Input: dimensioned drawing with shaded views. Units: mm. Origin: part minimum x, y, z. Round coordinates to 2 decimals unless told otherwise and drop trailing zeros. Order: outer loops, then holes, each group sorted by start corner. A loop starts at its lowest first (then second) coordinate and runs counter-clockwise, first axis right, second up. Notation, with made-up numbers: M 31.5,65.25 L 54.5,65.25 A9 ccw 54.5,79.25 Z; hole C 43,63 d9. An arc over 180 degrees is marked long. Answer as CSV lines item,"result". Start each with the question number.
Item 1: Line query: line 1 (Z direction, x = 5, y = 2.3); line 2 (X direction, y = 2.95, z = 3); line 3 (X direction, y = 6.5, z = 2.25). Output: solid intervals per line, ascending. Write a range as [from, to].
Item 2: First-contact query: P1, Ø1, axis at y = 5, z = 2.5, coming from the +X side. Flat tip, straight axial feed; report the tip coordinate or a pass-through.
Item 3: Section query B-B on y = 5. Return the cut outline in (x, z), plus the area to 3 significant figures.
Item 4: Section query D-D on z = 0.45. Return the cut outline in (x, y).
Item 5: Pull-direction query (Z, two-part tool) for the marked faces 1, 2 and 3; classes: +Z half, -Z half, draft (parallel to the pull), parting line (faces both ways), or undercut.
Item 6: Section query A-A on z = 3. Return the cut outline in (x, y).
Item 7: Section query C-C on x = 7. Return the cut outline in (y, z), plus the area to 3 significant figures.
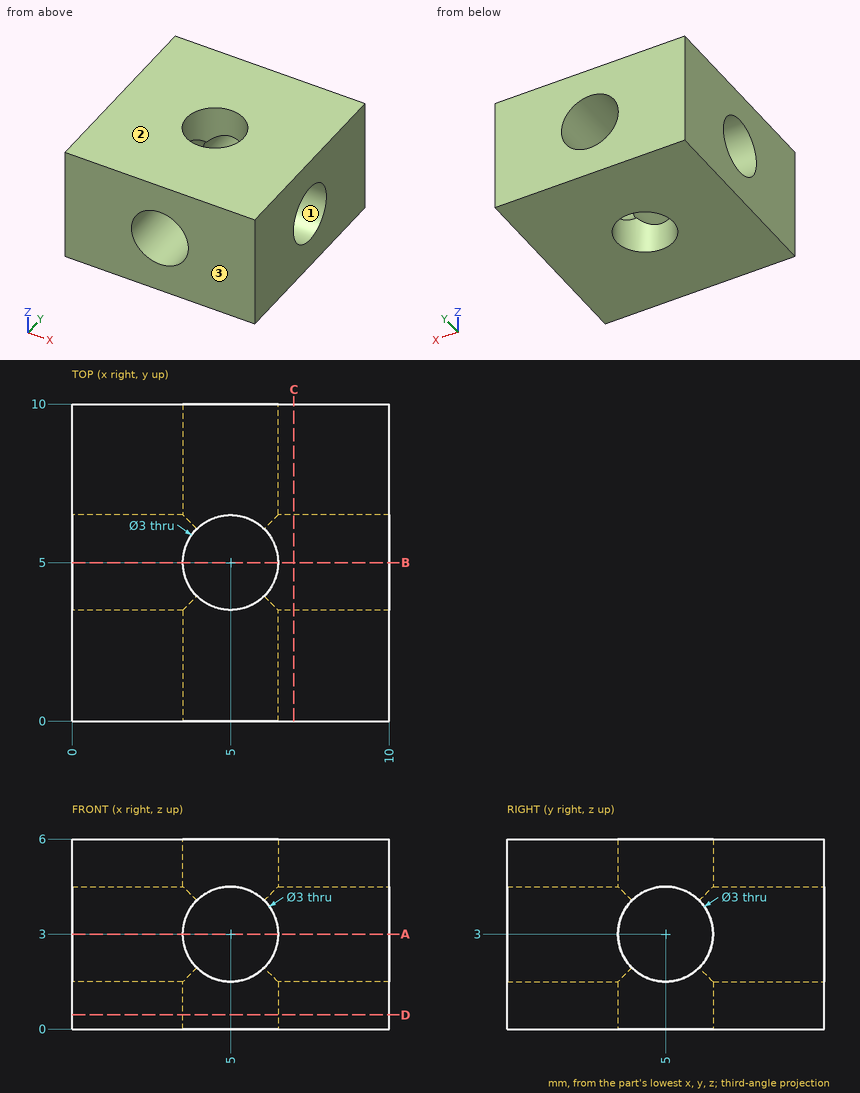
Results:
1,line 1,"[0, 1.5], [4.5, 6]"
1,line 2,"[0, 3.5], [6.5, 10]"
1,line 3,"[0, 3.7], [6.3, 10]"
2,P1,"through"
3,outline,"M 0,0 L 3.5,0 L 3.5,1.5 L 0,1.5 Z; M 0,4.5 L 3.5,4.5 L 3.5,6 L 0,6 Z; M 6.5,0 L 10,0 L 10,1.5 L 6.5,1.5 Z; M 6.5,4.5 L 10,4.5 L 10,6 L 6.5,6 Z"
3,area,"21.0 mm^2"
4,outline,"M 0,0 L 10,0 L 10,10 L 0,10 Z; hole C 5,5 d3"
5,face 1,"undercut"
5,face 2,"+Z half"
5,face 3,"draft"
6,outline,"M 0,0 L 3.5,0 L 3.5,3.5 L 0,3.5 Z; M 0,6.5 L 3.5,6.5 L 3.5,10 L 0,10 Z; M 6.5,0 L 10,0 L 10,3.5 L 6.5,3.5 Z; M 6.5,6.5 L 10,6.5 L 10,10 L 6.5,10 Z"
7,outline,"M 0,0 L 10,0 L 10,6 L 0,6 Z; hole C 5,3 d3"
7,area,"52.9 mm^2"
